Job drawing, mm, ordinate dimensions from the low corner. One solid piece. A direction names the side the tool comes from. Round coordinates to 2 decimals unless told otherwise and drop trailing zeros. Order: outer loops, then holes, each group sorted by start corner. A loop starts at its lowest first (then second) coordinate and runs counter-clockwise, first axis right, second up. Notation, with made-up numbers: (-17.5, -20.75) -> (16.5, -20.75) arc R9 ccw to (16.5, -8.75) -> close; hole circle Ø10 at (16, 39). An arc over 180 degrees is marked (long way). Return JSON: item names as keys, results as strings. Group by question number.
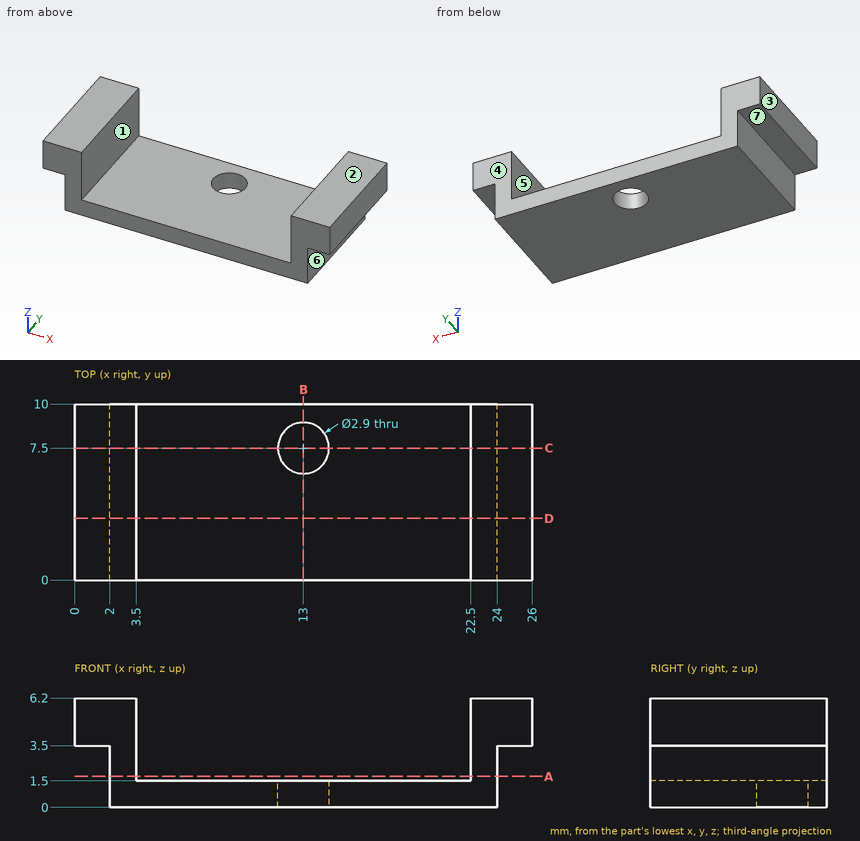
(1) Saw through at D-D, the plane y = 3.5. List the corners of the cut face in (x, z), and give its area (3 significant figures).
(2) Pin check, flat tip, straight feed: P1, Ø1.5, axis at y = 6.5, z = 2.5, coming from the +X side. Stop position of the tip, or through.
(3) Tool access for the marked faces 4, 5, 6 and 7: list every direction of +Z, -Z, +X, -X, +Y, -Y with a clear straight run to the whole face (end or side of a thin tool).
(4) Saw through at A-A, the plane z = 1.75. List the corners of the cut face in (x, y).
(5) Saw through at B-B, the plane x = 13. List the corners of the cut face in (y, z), and give its area (4 significant figures).
(6) Probe L1, parallel to Y at x = 13, z = 0.4; L2, parallel to X at y = 2, z = 4.5; L3, parallel to X at y = 5, z = 2.75. List the from-to ranges inside material, lowest first. Write a range as [from, to].
(7) Saw through at C-C, the plane y = 7.5. List the corners of the cut face in (x, z), and give its area (4 significant figures).
(8) Mould opens along X. For the marked faces 1, 2 and 3 say: pulls with the +X half, pulls with the -X half, needs draft (parallel to the pull), parting line crosses it, or undercut.
Results are:
{
 "1": {"outline": "(0, 3.5) -> (2, 3.5) -> (2, 0) -> (24, 0) -> (24, 3.5) -> (26, 3.5) -> (26, 6.2) -> (22.5, 6.2) -> (22.5, 1.5) -> (3.5, 1.5) -> (3.5, 6.2) -> (0, 6.2) -> close", "area": "57.9 mm^2"},
 "2": {"P1": "stops at x = 24"},
 "3": {"face 4": "+Z, -Z, +X, -X, +Y", "face 5": "+Z, +Y, -Y", "face 6": "-Z, +X, +Y, -Y", "face 7": "-Z, -X, +Y, -Y"},
 "4": {"outline": "(2, 0) -> (3.5, 0) -> (3.5, 10) -> (2, 10) -> close; (22.5, 0) -> (24, 0) -> (24, 10) -> (22.5, 10) -> close"},
 "5": {"outline": "(0, 0) -> (6.05, 0) -> (6.05, 1.5) -> (0, 1.5) -> close; (8.95, 0) -> (10, 0) -> (10, 1.5) -> (8.95, 1.5) -> close", "area": "10.65 mm^2"},
 "6": {"L1": "y = [0, 6.05], [8.95, 10]", "L2": "x = [0, 3.5], [22.5, 26]", "L3": "x = [2, 3.5], [22.5, 24]"},
 "7": {"outline": "(0, 3.5) -> (2, 3.5) -> (2, 0) -> (11.55, 0) -> (11.55, 1.5) -> (3.5, 1.5) -> (3.5, 6.2) -> (0, 6.2) -> close; (14.45, 0) -> (24, 0) -> (24, 3.5) -> (26, 3.5) -> (26, 6.2) -> (22.5, 6.2) -> (22.5, 1.5) -> (14.45, 1.5) -> close", "area": "53.55 mm^2"},
 "8": {"face 1": "undercut", "face 2": "needs draft", "face 3": "pulls with the -X half"}
}
